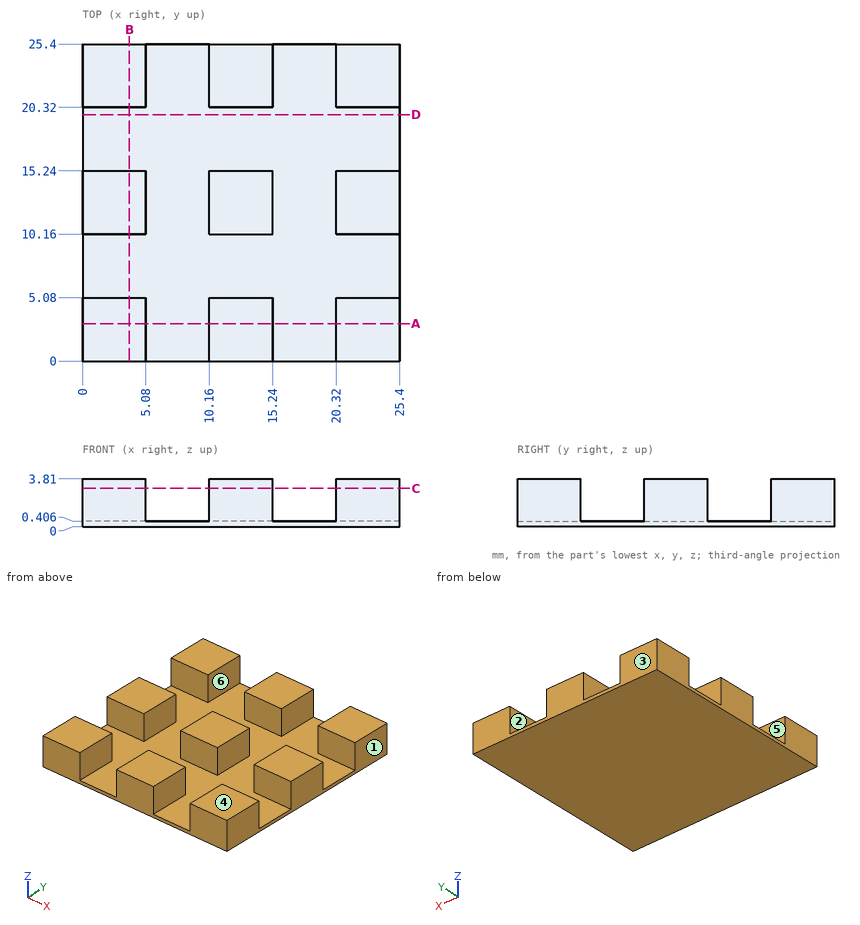
Geometry check sheet. Reference: drawing and pictorial views, mm from the part's lowest x, y, z. A direction names the side the tool comes from. Round coordinates to 2 decimals unless told otherwise and drop trailing zeros. Loops run counter-clockwise (first coordinate to the right, second up) from the corner with the lowest first, then second, coordinate; pieces in that order, holes last. Notation, with made-up numbers: (3, -3) - (55, -3) arc R10 ccw to (55, 8) - close; hole circle Ø5 at (-29, 32). An arc over 180 degrees is marked (long way). Write item = value, one per line. Start each with the question number.
Q1. Access from +Z, -Z, +X, -X, +Y, -Y to the whole of each face (thin tool, end or side, straight path). Record for the marked faces 4, 5 and 6.
Q2. Section check D-D (y = 19.75). Record the boundary of the cut face in (x, z).
Q3. Section check A-A (y = 3). Record the boundary of the cut face in (x, z).
Q4. Section check C-C (z = 3.05). Count the separate pieces of the cut face and the enclosed holes in it, plus the area to 3 significant figures.
Q5. Release check for a two-part mould opening along X. For the marked faces 1, 2 and 3 record: pulls with the +X half, pulls with the -X half, needs draft (parallel to the pull), parting line crosses it, or undercut.
Q6. Depth check by flat-ended pin: P1, Ø1.7, axis at y = 24, z = 1.5, coming from the -X side. Enter the tip coordinate at first touch or a pass-through.
Q7. Thickness scan on L1, parallel to X at y = 2, z = 0.85; L2, parallel to Z at x = 20, y = 21.5. Record the ranges inside material, lowest first.
Derived:
q1.face_4 = +Z, +X, -X, +Y, -Y
q1.face_5 = +Z, +X, -X
q1.face_6 = +Z, +Y, -Y
q2.outline = (0, 0) - (25.4, 0) - (25.4, 0.41) - (0, 0.41) - close
q3.outline = (0, 0) - (25.4, 0) - (25.4, 3.81) - (20.32, 3.81) - (20.32, 0.41) - (15.24, 0.41) - (15.24, 3.81) - (10.16, 3.81) - (10.16, 0.41) - (5.08, 0.41) - (5.08, 3.81) - (0, 3.81) - close
q4.separate_pieces = 9
q4.enclosed_holes = 0
q4.area = 232 mm^2
q5.face_1 = pulls with the +X half
q5.face_2 = undercut
q5.face_3 = needs draft
q6.P1 = 0
q7.L1 = 0 to 5.08, 10.16 to 15.24, 20.32 to 25.4
q7.L2 = 0 to 0.41
